from build123d import *

# Parameters (mm, degrees)
F0_R        = 12.7
F0_R_2      = 2.2479
F1_DEPTH    = 6.35
F2_W        = 7.9375
F2_H        = 7.9375
F2_R        = 2.2479
F3_DEPTH    = 7.9375
F5_REACH    = 20.5318866107
F6_T1_DEPTH = 17.859375
F7_W        = 1.5875
F7_H        = 3.175
F8_DEPTH    = 6.35
F9_COUNT    = 20
F9_ANGLE    = 342


# Not quite as in the source:
# - a fillet or chamfer that OpenCascade refuses, or shapes differently, is made with other operations: its cross-section is extruded or revolved along the edge and cut away or added


with BuildPart() as f1:
    # F0 (on Top) → F1 (new body)
    with BuildSketch(Plane.XY):
        Circle(F0_R)
        Circle(F0_R_2, mode=Mode.SUBTRACT)
    extrude(amount=F1_DEPTH)

    # F2 (on face) → F3 (join)
    with BuildSketch(Plane(origin=(0, 0, 0), x_dir=(1, 0, 0), z_dir=(0, 0, -1))):
        Rectangle(F2_W, F2_H)
        Circle(F2_R, mode=Mode.SUBTRACT)
    extrude(amount=F3_DEPTH)

    f5_end = f1.faces().sort_by_distance((-2.2479, 0, -0.79375))[0]
    # F4 (on face) → F5 (cut, up to a face of the model that its end follows)
    with BuildSketch(Plane.YZ.offset(3.96875)):
        with BuildLine():
            ThreePointArc((-1.7272, -3.96875), (0, -5.69595), (1.7272, -3.96875))
            Line((1.7272, -3.96875), (-1.7272, -3.96875))
        make_face()
        with BuildLine():
            Line((-1.7272, -3.96875), (1.7272, -3.96875))
            ThreePointArc((1.7272, -3.96875), (0, -2.24155), (-1.7272, -3.96875))
        make_face()
    f5_long = extrude(amount=-F5_REACH, mode=Mode.PRIVATE)
    add(split(f5_long, bisect_by=f5_end, keep=Keep.ALL, mode=Mode.PRIVATE).solids().sort_by_distance((3.96875, 0, -3.96875))[0], mode=Mode.SUBTRACT)

    # F6: fillet of radius 3.96875 on 4 edges, made by hand

    # F6_s2 → F6_t1 (cut)
    with BuildSketch(Plane.XY.offset(-17.859375)):
        with BuildLine():
            ThreePointArc((0, 3.96875), (2.8063300378, 2.8063300378), (3.96875, 0))
            Line((3.96875, 0), (3.96875, 3.96875))
            Line((3.96875, 3.96875), (0, 3.96875))
        make_face()
        with BuildLine():
            ThreePointArc((0, 3.96875), (-2.8063300378, 2.8063300378), (-3.96875, 0))
            Line((-3.96875, 0), (-3.96875, 3.96875))
            Line((-3.96875, 3.96875), (0, 3.96875))
        make_face()
        with BuildLine():
            ThreePointArc((-3.96875, 0), (-2.8063300378, -2.8063300378), (0, -3.96875))
            Line((0, -3.96875), (-3.96875, -3.96875))
            Line((-3.96875, -3.96875), (-3.96875, 0))
        make_face()
        with BuildLine():
            ThreePointArc((0, -3.96875), (2.8063300378, -2.8063300378), (3.96875, 0))
            Line((3.96875, 0), (3.96875, -3.96875))
            Line((3.96875, -3.96875), (0, -3.96875))
        make_face()
    extrude(amount=F6_T1_DEPTH, mode=Mode.SUBTRACT)

    # F7 (on face) → F8 (join, through all)
    with BuildSketch(Plane.XY.offset(6.35)):
        with Locations((13.3941406189, 0)):
            Rectangle(F7_W, F7_H)
    f8 = extrude(amount=-F8_DEPTH)

    # F9: F8 ×20 about axis
    f9_axis = Axis((0, 0, 0), (0, 0, -1))
    for i in range(1, F9_COUNT):
        add(f8.rotate(f9_axis, i * F9_ANGLE / (F9_COUNT - 1)))


solid = f1.part
CAD build for the part. Positions are in the model's coordinates, mm. A direction names the side the tool comes from. Coordinates: 2 decimals unless noted, no trailing zeros. Write each loop counter-clockwise with the first axis right and the second up, starting at its lowest first coordinate (ties: lowest second). Pieces come first, ordered by that corner, then holes. Notation, with made-up numbers: M -32.5,-21 L -18.5,-21 A27 cw -18.5,-2 Z; hole C -31,-12 d11. An arc over 180 degrees is marked long. Answer as a JSON object with one key per item and string values. Group by question number.
1) Saw through at B-B (y = -1). Write the cut outline in (x, z).
2) Saw through at A-A (z = -1.75). Write the cut outline in (x, y), plus the area to 3 significant figures.
3) Mould opens along X. For faces 6 (the face through (13.219, 2.626, 3.219)), 7 (the face through (-2.246, -0.099, -0.694)), 8 (the face through (3, 3, 0)) say: +X half, -X half, draft (parallel to the pull), parting line (faces both ways), or undercut.
4) Wall check: line 1 (Z direction, x = 2.8, y = 0); line 2 (Y direction, x = 0, z = 0.75); line 3 (X direction, y = 0, z = -1). Give the ranges that are in metal, low to high. Write a range as from..to.
5) Pin check, flat tips, straight feed: pin 1 Ø3 at (x, z) = (-7.5, 4.5) entering from -Y; pin 2 Ø3 at (y, z) = (0, -3.97) entering from -X; pin 3 Ø0.8 at (y, z) = (13, 1.5) entering from +X. Stop position of each tip, or through.
6) Tool access for faces 1 (the face through (9.15, -9.89, 3.22)), 2 (the face through (13, -1.588, 3)), 3 (the face through (-6.58, 11.76, 3.22)), 4 (the face through (2.626, -13.219, 3.219)), 5 (the face through (-13, 1.587, 3)): list every direction of +Z, -Z, +X, -X, +Y, -Y with a clear straight run to the whole face (end or side of a thin tool).
Values follow:
{
 "1": {"outline": "M -14.19,0 L -3.84,0 L -3.84,-7.94 L -2.01,-7.94 L -2.01,6.35 L -14.19,6.35 Z; M 2.01,-7.94 L 3.84,-7.94 L 3.84,-5.38 L 2.01,-5.38 Z; M 2.01,-2.56 L 3.84,-2.56 L 3.84,0 L 14.19,0 L 14.19,6.35 L 2.01,6.35 Z"},
 "2": {"outline": "C 0,0 d7.94; hole C 0,0 d4.5", "area": "33.6 mm2"},
 "3": {"face 6": "+X half", "face 7": "undercut", "face 8": "draft"},
 "4": {"line 1": "z = -7.94..-5.7, -2.24..6.35", "line 2": "y = -14.19..-2.25, 2.25..14.19", "line 3": "x = -3.97..-2.25, 2.25..3.97"},
 "5": {"pin 1": "stops at y = -12.41", "pin 2": "stops at x = -3.97", "pin 3": "stops at x = 5.89"},
 "6": {"face 1": "+Z, -Z", "face 2": "+Z, -Z, +X", "face 3": "+Z, -Z, +Y", "face 4": "+Z, -Z, -Y", "face 5": "+Z, -Z, -X"}
}
